Design review of the part shown in the three views and the two pictorial views. Dimensions are in mm from the part's minimum x, y and z. A direction names the side the tool comes from. Give positions to 0.01 mm unless a question says otherwise; leave off trailing zeros. Order: outer loops, then holes, each group sorted by start corner. A loop starts at its lowest first (then second) coordinate and runs counter-clockwise, first axis right, second up.
Item 1: The part is to be moulded in two halves that separate along Y. For the marked faces 4, 5, 6 and 7, say which applies: released by +Y, released by -Y, zero draft, split by the parting line, or undercut.
Item 2: Consider section A-A (y = 9). Give the boundary of the cut face in (x, z).
Item 3: For probe 1 along X at (y, z) = (10, 52); probe 2 along X at (y, z) = (62.5, 18); probe 3 along Y at (x, z) = (53, 29) (1 decimal), list the stretches that pass through material, from the lowest coordinate up.
Item 4: Machinability: for the marked faces 1, 2 and 3, which of the approach directions +Z, -Z, +X, -X, +Y, -Y give a long, thin tool a straight path to every point of the face, cutting with its end or side? Answer none if there is none.
Item 5: Consider section C-C (z = 10.5). Give the boundary of the cut face in (x, y) (1 decimal).
Item 6: For P1, Ø2, axis at x = 88.5, z = 52.5, coming from the +Y side; P2, Ø4, axis at y = 64.5, z = 41, coming from the +X side; P3, Ø5.5, axis at x = 43, z = 47.5, coming from the -Y side (1 decimal), all flat-tipped, find the tip position at first contact; note any pin that passes through.
Item 7: Consider section D-D (x = 21). Give the boundary of the cut face in (y, z) (1 decimal), plus the area to 3 significant figures.
Item 8: Consider section B-B (x = 45.5). Give the boundary of the cut face in (y, z) (1 decimal).
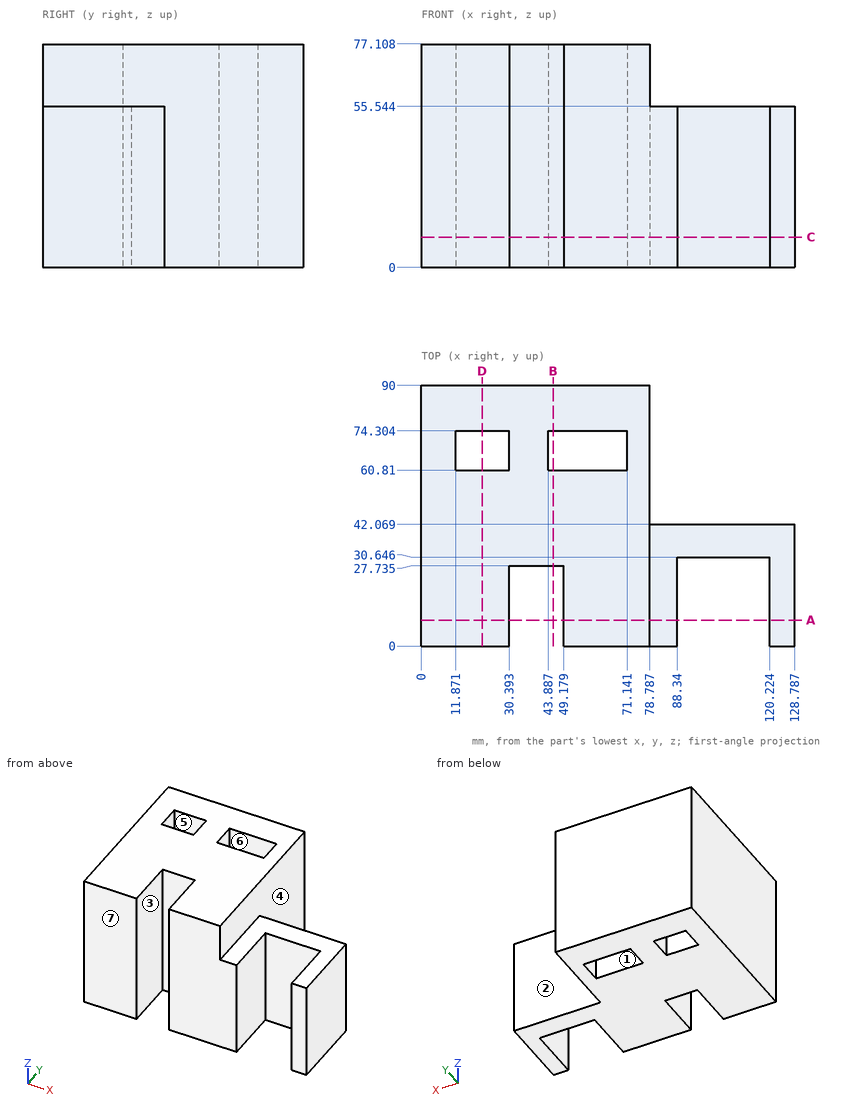
Resolved:
1. face 4: zero draft
1. face 5: undercut
1. face 6: undercut
1. face 7: released by -Y
2. outline: (0, 0) - (30.39, 0) - (30.39, 77.11) - (0, 77.11) - close; (49.18, 0) - (88.34, 0) - (88.34, 55.54) - (78.79, 55.54) - (78.79, 77.11) - (49.18, 77.11) - close; (120.22, 0) - (128.79, 0) - (128.79, 55.54) - (120.22, 55.54) - close
3. probe 1: x = 0 to 30.39, 49.18 to 88.34, 120.22 to 128.79
3. probe 2: x = 0 to 11.87, 30.39 to 43.89, 71.14 to 78.79
3. probe 3: y = 0 to 60.8, 74.3 to 90
4. face 1: +Z, -Z
4. face 2: +Z, -Z, +X, +Y
4. face 3: +Z, -Z, -Y
5. outline: (0, 0) - (30.4, 0) - (30.4, 27.7) - (49.2, 27.7) - (49.2, 0) - (88.3, 0) - (88.3, 30.6) - (120.2, 30.6) - (120.2, 0) - (128.8, 0) - (128.8, 42.1) - (78.8, 42.1) - (78.8, 90) - (0, 90) - close; hole (11.9, 60.8) - (30.4, 60.8) - (30.4, 74.3) - (11.9, 74.3) - close; hole (43.9, 60.8) - (71.1, 60.8) - (71.1, 74.3) - (43.9, 74.3) - close
6. P1: stops at y = 42.07
6. P2: stops at x = 78.79
6. P3: stops at y = 27.7
7. outline: (0, 0) - (60.8, 0) - (60.8, 77.1) - (0, 77.1) - close; (74.3, 0) - (90, 0) - (90, 77.1) - (74.3, 77.1) - close
7. area: 5,900 mm2
8. outline: (27.7, 0) - (60.8, 0) - (60.8, 77.1) - (27.7, 77.1) - close; (74.3, 0) - (90, 0) - (90, 77.1) - (74.3, 77.1) - close
